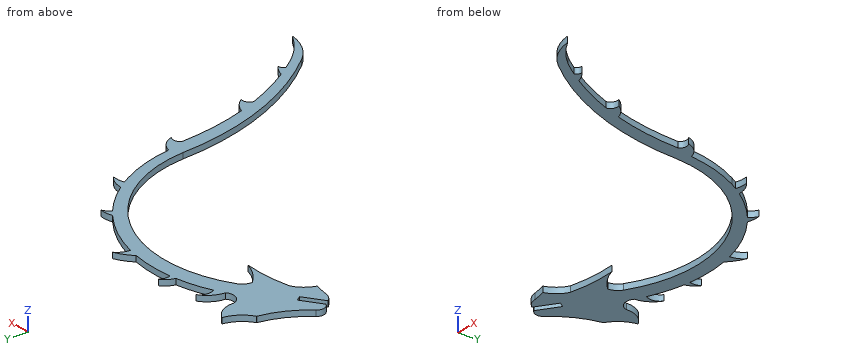
from build123d import *

# Parameters (mm, degrees)
BOSS_EXTRUDE1_DEPTH = 1.524


with BuildPart() as part:
    # Sketch1 → Boss-Extrude1 (new body)
    with BuildSketch(Plane.XY):
        with BuildLine():
            Line((-39.117691612, 31.705702494), (-34.035061267, 35.245462587))
            Line((-34.035061267, 35.245462587), (-34.907334502, 36.4982372))
            Line((-34.907334502, 36.4982372), (-39.989964847, 32.957484201))
            ThreePointArc((-39.989964847, 32.957484201), (-41.156381442, 34.371130843), (-40.72943499, 36.153444291))
            ThreePointArc((-40.72943499, 36.153444291), (-37.157257908, 41.392315435), (-35.149645056, 47.406940162))
            ThreePointArc((-35.149645056, 47.406940162), (-35.150000593, 47.436618983), (-35.150119107, 47.466299697))
            ThreePointArc((-35.150119107, 47.466299697), (-32.474220558, 50.029100651), (-31.092386734, 53.46696584))
            ThreePointArc((-31.092386734, 53.46696584), (-28.528895289, 51.083388449), (-27.722652605, 47.677085129))
            ThreePointArc((-27.722652605, 47.677085129), (-25.864549179, 45.627042683), (-23.153757297, 46.180964831))
            ThreePointArc((-23.153757297, 46.180964831), (-22.178534836, 49.206145698), (-19.954812919, 51.477233316))
            ThreePointArc((-19.954812919, 51.477233316), (-21.130091376, 49.619411518), (-20.702707555, 47.462996819))
            ThreePointArc((-20.702707555, 47.462996819), (-16.368548246, 49.204688548), (-11.850579294, 50.390598976))
            ThreePointArc((-11.850579294, 50.390598976), (-11.153919, 52.10102423), (-9.892322836, 53.449825638))
            ThreePointArc((-9.892322836, 53.449825638), (-10.390962499, 52.098435339), (-10.305463017, 50.66052467))
            ThreePointArc((-10.305463017, 50.66052467), (-4.659496824, 51.089737509), (0.986334207, 50.658750415))
            ThreePointArc((0.986334207, 50.658750415), (2.931593893, 52.336657489), (5.181027531, 53.577405529))
            ThreePointArc((5.181027531, 53.577405529), (4.013781328, 52.043650888), (3.542618472, 50.174728054))
            ThreePointArc((3.542618472, 50.174728054), (10.941086412, 47.665032068), (17.653861509, 43.668214296))
            ThreePointArc((17.653861509, 43.668214296), (19.271772807, 44.086118721), (20.942706276, 44.069919276))
            ThreePointArc((20.942706276, 44.069919276), (19.933918295, 43.40682582), (19.151343007, 42.48762941))
            ThreePointArc((19.151343007, 42.48762941), (22.950326986, 38.849120016), (26.199236503, 34.712017549))
            ThreePointArc((26.199236503, 34.712017549), (28.587130465, 34.336897034), (30.651629038, 33.079678433))
            ThreePointArc((30.651629038, 33.079678433), (29.023098561, 33.126789379), (27.436671978, 32.755869369))
            ThreePointArc((27.436671978, 32.755869369), (27.926256891, 31.900308765), (28.393045297, 31.032100312))
            ThreePointArc((28.393045297, 31.032100312), (31.169330508, 24.1759064), (32.596114117, 16.917845842))
            ThreePointArc((32.596114117, 16.917845842), (35.116195442, 15.563753706), (36.545589929, 13.085607866))
            ThreePointArc((36.545589929, 13.085607866), (34.988216261, 13.405663895), (33.766569049, 12.388104711))
            ThreePointArc((33.766569049, 12.388104711), (34.557842987, 3.332770711), (36.545589929, -5.537068656))
            ThreePointArc((36.545589929, -5.537068656), (38.757623722, -6.672814151), (40.411337246, -8.52975866))
            ThreePointArc((40.411337246, -8.52975866), (38.887733864, -8.706049408), (38.022049175, -9.972159875))
            ThreePointArc((38.022049175, -9.972159875), (40.611583977, -16.03077135), (43.773329776, -21.811413788))
            ThreePointArc((43.773329776, -21.811413788), (45.465168408, -22.463416845), (46.96111524, -23.487901602))
            ThreePointArc((46.96111524, -23.487901602), (46.009909008, -23.664428409), (45.493072894, -24.482252008))
            ThreePointArc((45.493072894, -24.482252008), (46.778816766, -26.31501847), (48.123987434, -28.104623476))
            ThreePointArc((48.123987434, -28.104623476), (51.40918984, -31.384637985), (55.283874059, -33.941564308))
            ThreePointArc((55.283874059, -33.941564308), (50.301959018, -32.513729239), (46.276855411, -29.249264289))
            ThreePointArc((46.276855411, -29.249264289), (34.30827338, -8.358491308), (29.894604694, 15.309860564))
            ThreePointArc((29.894604694, 15.309860564), (11.897133565, 43.455618791), (-21.477635315, 41.96649978))
            ThreePointArc((-21.477635315, 41.96649978), (-22.656445953, 40.735662089), (-23.136633245, 39.10043241))
            ThreePointArc((-23.136633245, 39.10043241), (-20.241057696, 36.637371423), (-16.767124999, 35.093733251))
            ThreePointArc((-16.767124999, 35.093733251), (-22.9849523, 34.969630573), (-29.11414449, 33.916169174))
            ThreePointArc((-29.11414449, 33.916169174), (-31.355074443, 32.068657032), (-32.706500842, 29.497914951))
            ThreePointArc((-32.706500842, 29.497914951), (-34.36207957, 29.840980807), (-36.03028603, 30.116157682))
            ThreePointArc((-36.03028603, 30.116157682), (-37.766569844, 30.536876005), (-39.117691612, 31.705702494))
        make_face()
    extrude(amount=BOSS_EXTRUDE1_DEPTH)


solid = part.part
The model under review builds one solid part; all positions refer to its coordinate system, in mm. Coordinates: 2 decimals unless noted, no trailing zeros. Loops run counter-clockwise (first coordinate to the right, second up) from the corner with the lowest first, then second, coordinate; pieces in that order, holes last.
(1) Consider section C-C, the plane y = -4. Give the boundary of the cut face in (x, z), plus the area to 3 significant figures.
Determined:
outline: (32.86, 0) - (36.11, 0) - (36.11, 1.52) - (32.86, 1.52) - close
area: 4.95 mm2
(2) Consider section A-A, the plane y = 40.5. Give the boundary of the cut face in (x, z), plus the area to 3 significant figures.
Determined:
outline: (-37.62, 0) - (-22.78, 0) - (-22.78, 1.52) - (-37.62, 1.52) - close; (16.59, 0) - (21.36, 0) - (21.36, 1.52) - (16.59, 1.52) - close
area: 29.9 mm2
(3) Consider section B-B, the plane x = 15. Give the boundary of the cut face in (y, z).
Determined:
outline: (41.63, 0) - (45.48, 0) - (45.48, 1.52) - (41.63, 1.52) - close
(4) Wall thickness on L1, parallel to X at y = 37, z = 1.3; L2, parallel to X at y = -25.5, z = 0.9; L3, parallel to Y at x = 21, z = 0.25: over which ranges is each line inside the solid? List them lowest first.
Determined:
L1: x = -40 to -20.79, 20.55 to 24.52
L2: x = 43.39 to 46.2
L3: y = 36.53 to 40.85
